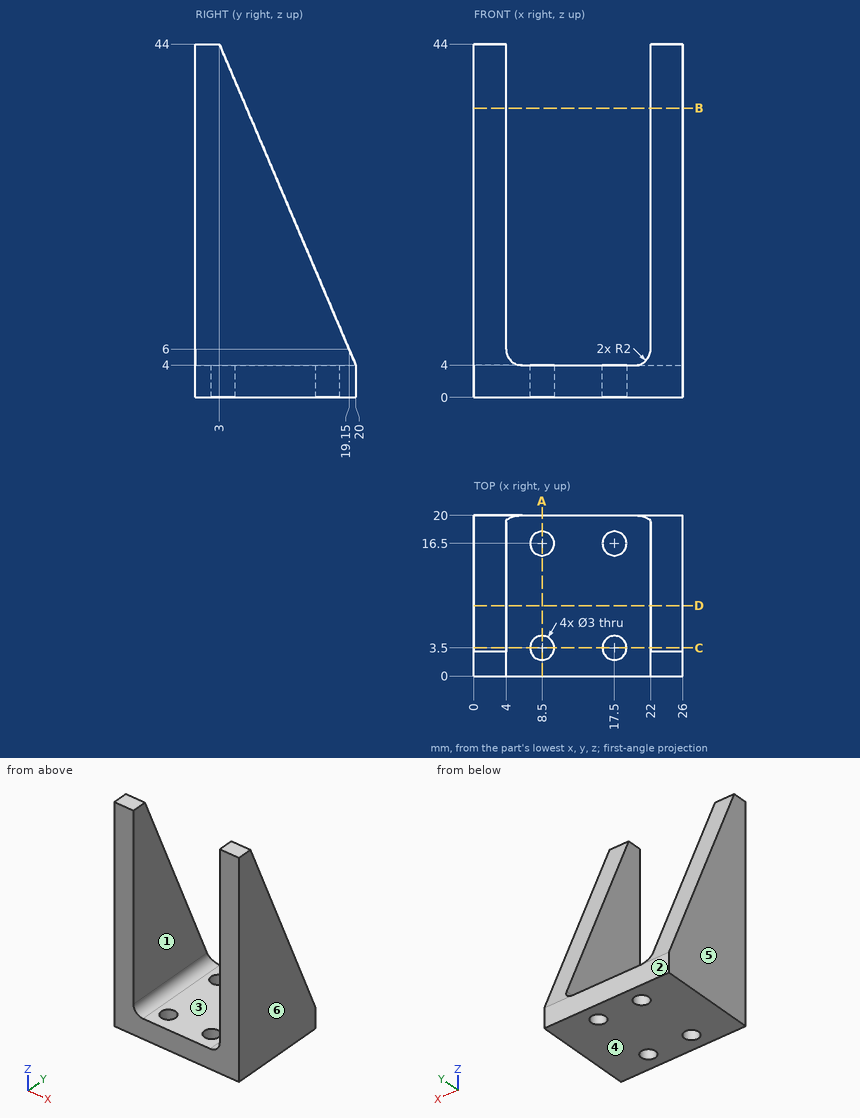
Check sheet for the drawn part. Datum: minimum x, y, z corner. Units: mm. A direction names the side the tool comes from. Coordinates: 2 decimals unless noted, no trailing zeros. Write each loop counter-clockwise with the first axis right and the second up, starting at its lowest first coordinate (ties: lowest second). Pieces come first, ordered by that corner, then holes. Notation, with made-up numbers: M 76.25,-1.5 L 88.25,-1.5 A17 ccw 88.25,18.5 Z; hole C 75.5,60 d5. An arc over 180 degrees is marked long. One line per item, written item: value.
Item 1: Section check A-A, the plane x = 8.5. Record the boundary of the cut face in (y, z), plus the area to 3 significant figures.
Check sheet entries:
outline: M 0,0 L 2,0 L 2,4 L 0,4 Z; M 5,0 L 15,0 L 15,4 L 5,4 Z; M 18,0 L 20,0 L 20,4 L 18,4 Z
area: 56.0 mm^2
Item 2: Section check C-C, the plane y = 3.5. Record the boundary of the cut face in (x, z).
Check sheet entries:
outline: M 0,0 L 7,0 L 7,4 L 6,4 A2 cw 4,6 L 4,42.82 L 0,42.82 Z; M 10,0 L 16,0 L 16,4 L 10,4 Z; M 19,0 L 26,0 L 26,42.82 L 22,42.82 L 22,6 A2 cw 20,4 L 19,4 Z
Item 3: Section check D-D, the plane y = 8.75. Record the boundary of the cut face in (x, z), plus the area to 3 significant figures.
Check sheet entries:
outline: M 0,0 L 26,0 L 26,30.47 L 22,30.47 L 22,6 A2 cw 20,4 L 6,4 A2 cw 4,6 L 4,30.47 L 0,30.47 Z
area: 317 mm^2
Item 4: Mould release check, pull along X, two halves, no side actions. Record for the marked faces 3, 4, 5 and 6: pulls with the +X half, pulls with the -X half, needs draft (parallel to the pull), parting line crosses it, or undercut.
Check sheet entries:
face 3: undercut
face 4: needs draft
face 5: pulls with the -X half
face 6: pulls with the +X half
Item 5: Section check B-B, the plane z = 36. Record the boundary of the cut face in (x, y).
Check sheet entries:
outline: M 0,0 L 4,0 L 4,6.4 L 0,6.4 Z; M 22,0 L 26,0 L 26,6.4 L 22,6.4 Z
Item 6: Access from +Z, -Z, +X, -X, +Y, -Y to the whole of each face (thin tool, end or side, straight path). Record for the marked faces 1 and 2.
Check sheet entries:
face 1: +Z, +Y, -Y
face 2: +Z, -Z, +X, -X, +Y
Item 7: Scan lines: line 1 along Y through (x, z) = (17.5, 1.5); line 2 along X through (y, z) = (7.5, 33); line 3 along Z through (x, y) = (6, 15.75). Record each from-to range of solid material in increasing order.
Check sheet entries:
line 1: y = 0 to 2, 5 to 15, 18 to 20
line 2: x = 0 to 4, 22 to 26
line 3: z = 0 to 4
Item 8: Gauge pin test, flat ends, axial feed: pin 1 Ø9.5 at (y, z) = (12.5, 32.5) entering from +X; pin 2 Ø11 at (x, y) = (11.5, 11.5) entering from +Z; pin 3 Ø3 at (x, z) = (6, 26) entering from -Y. Record the tip position at first contact, or that the pin passes through.
Check sheet entries:
pin 1: stops at x = 26
pin 2: stops at z = 4
pin 3: passes through
